Study the drawing (mm; zero at the part's minimum x, y, z) and answer. A direction names the side the tool comes from. Give positions to 0.01 mm unless a question says otherwise; leave off trailing zeros. Write each loop counter-clockwise with the first axis right and the second up, starting at its lowest first coordinate (ties: lowest second). Pieces come first, ordered by that corner, then holes. Notation, with made-up numbers: (46, 20.5) -> (74, 20.5) arc R12 cw to (74, 33.5) -> close; hole circle Ø7 at (67, -37). An arc over 180 degrees is marked (long way). One line per question, with ' | ' between items.
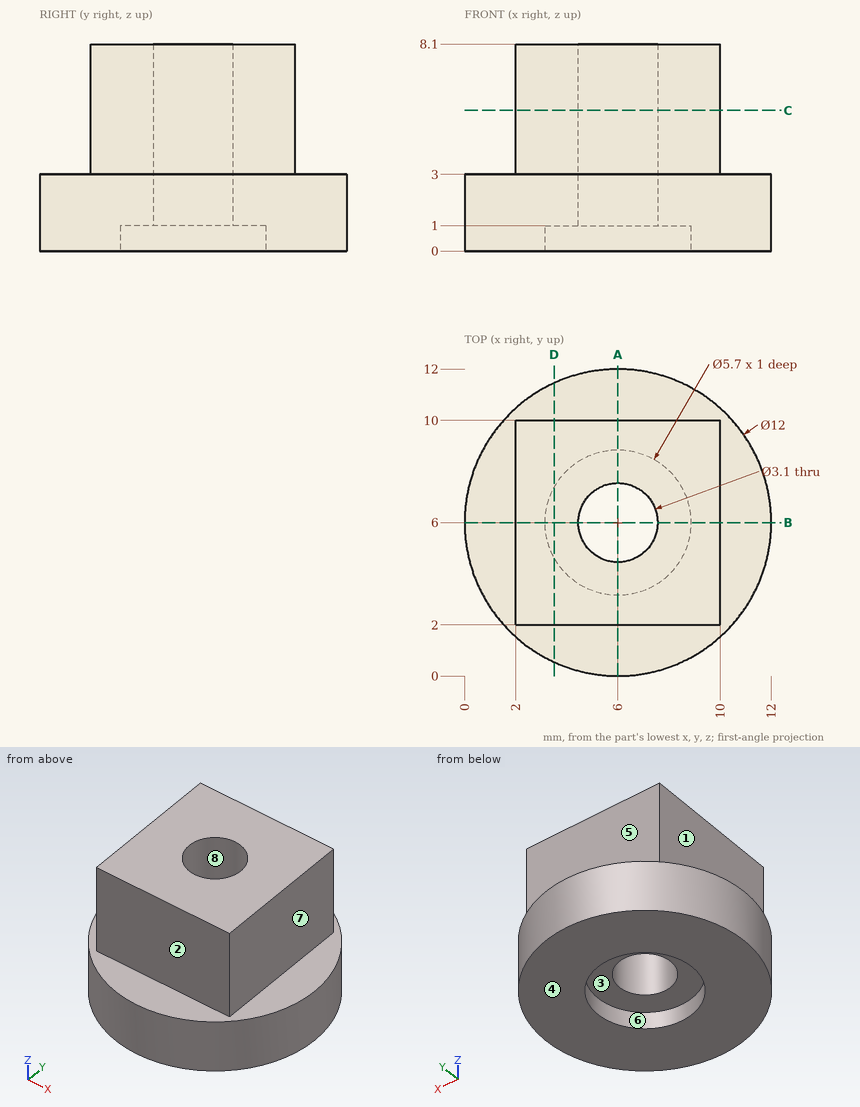
Item 1: Find section A-A (x = 6). Write down the section's boundary in (y, z).
Answers below:
outline: (0, 0) -> (3.15, 0) -> (3.15, 1) -> (4.45, 1) -> (4.45, 8.1) -> (2, 8.1) -> (2, 3) -> (0, 3) -> close; (7.55, 1) -> (8.85, 1) -> (8.85, 0) -> (12, 0) -> (12, 3) -> (10, 3) -> (10, 8.1) -> (7.55, 8.1) -> close
Item 2: A tool of negligible diameter and unlimited length cuts with its end or side. For the marked faces 4, 5, 6, 7 and 8, from which of +Z, -Z, +X, -X, +Y, -Y can it reach the whole face along a straight path? Write none if from no direction.
Answers below:
face 4: -Z, +X, -X, +Y, -Y | face 5: +Z, +X, -X, +Y | face 6: -Z | face 7: +Z, +X, +Y, -Y | face 8: +Z, -Z
Item 3: Consider line 1 (Y direction, x = 6, z = 4.5); line 2 (Y direction, x = 6, z = 0.7); line 3 (Z direction, x = 6.75, y = 7.5). Determine where each line is inside the solid, lowest interval first. Write a range as [from, to].
Answers below:
line 1: [2, 4.45], [7.55, 10] | line 2: [0, 3.15], [8.85, 12] | line 3: [1, 8.1]
Item 4: Find section C-C (z = 5.5). Write down the section's boundary in (x, y), then the cut area to 3 significant figures.
Answers below:
outline: (2, 2) -> (10, 2) -> (10, 10) -> (2, 10) -> close; hole circle Ø3.1 at (6, 6) | area: 56.5 mm²
Item 5: Determine the mould class of the marked faces 1, 2 and 3 for opening direction Y: pulls with the +Y half, pulls with the -Y half, needs draft (parallel to the pull), parting line crosses it, or undercut.
Answers below:
face 1: needs draft | face 2: pulls with the -Y half | face 3: undercut
Item 6: Flat-ended cylindrical pins translate along their axes: pin 1 (1.5 mm diameter, centred on x = 7, z = 5, fed in from -Y); pin 2 (1.5 mm diameter, centred on y = 7.5, z = 7, fed in from -X); pin 3 (4 mm diameter, centred on y = 5.5, z = 5.5, fed in from +X). Find the tip coordinate at first contact, or state that the pin passes through.
Answers below:
pin 1: y = 2 | pin 2: x = 2 | pin 3: x = 10
Item 7: Find section D-D (x = 3.5). Write down the section's boundary in (y, z).
Answers below:
outline: (0.55, 0) -> (4.63, 0) -> (4.63, 1) -> (7.37, 1) -> (7.37, 0) -> (11.45, 0) -> (11.45, 3) -> (10, 3) -> (10, 8.1) -> (2, 8.1) -> (2, 3) -> (0.55, 3) -> close
